Check sheet for the modelled part. Datum: model origin and axes. Units: mm. A direction names the side the tool comes from. Round coordinates to 2 decimals unless told otherwise and drop trailing zeros. Order: outer loops, then holes, each group sorted by start corner. A loop starts at its lowest first (then second) coordinate and runs counter-clockwise, first axis right, second up.
(1) Thickness scan on probe 1 along Y at (x, z) = (6.25, 8); probe 2 along Y at (x, z) = (-6.25, 5); probe 3 along X at (y, z) = (1, 5.75). Record the ranges inside material, lowest first.
(2) Mould release check, pull along Y, two halves, no side actions. Record for faces 1 (the cylindrical face through (11.25, -0.11, 8.73)), 2 (the cylindrical face through (-7.837, -1.217, 5.035)), 3 (the flat face through (3.8, 2.3, 7.5)): released by +Y, released by -Y, zero draft, split by the parting line, or undercut.
(3) Sectioned sample at D-D, the plane x = -1.5. Enter the section's corners in (y, z), and give its area (3 significant figures).
(4) Sectioned sample at C-C, the plane y = 3.75. Enter the section's corners in (x, z), and give its area (4 significant figures).
(5) Depth check by flat-ended pin: pin 1 (3.5 mm diameter, centred on x = 6.25, y = 0, fed in from -Z); pin 2 (1 mm diameter, centred on x = 8.5, y = -3.5, fed in from -Z); pin 3 (3 mm diameter, centred on y = 1.5, z = 1.5, fed in from -X); pin 4 (5 mm diameter, centred on x = 3.5, y = -1, fed in from -Z). Enter the tip coordinate at first touch or a pass-through.
(6) Sectioned sample at A-A, the plane y = 0. Enter the section's corners in (x, z), and give its area (3 significant figures).
(7) Sectioned sample at B-B, the plane z = 3.25. Enter the section's corners in (x, y), and give its area (3 significant figures).
(8) Tool access check on faces 4 (the flat face through (1.05, 0, 4)), 5 (the flat face through (-4, 0, 2.5)), 6 (the flat face through (-1.028, 0, 9)). Record the directions out of +Z, -Z, +X, -X, +Y, -Y that give a thin tool (end or side, any length) a straight path to the whole face; none if there is none.
```python
from build123d import *

# Parameters (mm, degrees)
EXTRUDE_1_DEPTH     = 10
SKETCH_3_W          = 5
SKETCH_3_H          = 2.5
CUT_EXTRUDE_2_DEPTH = 19.071040369
SKETCH_4_W          = 10.2
SKETCH_4_H          = 2.5
SKETCH_4_W_2        = 10.22157303
SKETCH_4_H_2        = 7.5
CUT_EXTRUDE_3_DEPTH = 19.071040369
EXTRUDE_START       = -1.5
SKETCH_2_R          = 2
EXTRUDE_2_DEPTH     = 3
SKETCH_2_3_R        = 3.1
SKETCH_2_3_R_2      = 2
CUT_EXTRUDE_4_DEPTH = 16.860721926


with BuildPart() as part:
    # Sketch 1 → Extrude 1 (new body)
    with BuildSketch(Plane.XY):
        with BuildLine():
            Line((-6.25, -5), (6.25, -5))
            ThreePointArc((6.25, -5), (11.25, 0), (6.25, 5))
            Line((6.25, 5), (-6.25, 5))
            ThreePointArc((-6.25, 5), (-11.25, 0), (-6.25, -5))
        make_face()
    extrude(amount=EXTRUDE_1_DEPTH)

    # Sketch 3 → Cut-Extrude 2 (cut, through all)
    with BuildSketch(Plane(origin=(0, 5, 0), x_dir=(1, 0, 0), z_dir=(0, 1, 0))):
        with Locations((8.75, -5)):
            Rectangle(SKETCH_3_W, SKETCH_3_H)
    extrude(amount=-CUT_EXTRUDE_2_DEPTH, mode=Mode.SUBTRACT)

    # Sketch 4 → Cut-Extrude 3 (cut, through all)
    with BuildSketch(Plane(origin=(0, 5, 0), x_dir=(1, 0, 0), z_dir=(0, 1, 0))):
        with Locations((-6.15, -1.25)):
            Rectangle(SKETCH_4_W, SKETCH_4_H)
        with Locations((-6.139213485, -8.75)):
            Rectangle(SKETCH_4_W_2, SKETCH_4_H)
        with Locations((6.15, -3.75)):
            Rectangle(SKETCH_4_W, SKETCH_4_H_2)
    extrude(amount=-CUT_EXTRUDE_3_DEPTH, mode=Mode.SUBTRACT)

    # Sketch 2 → Extrude 2 (add)
    with BuildSketch(Plane.XY.offset(10).offset(EXTRUDE_START)):
        with Locations((-6.25, 0)):
            Circle(SKETCH_2_R)
    extrude(amount=-EXTRUDE_2_DEPTH)

    # Sketch 2_3 → Cut-Extrude 4 (cut, through all)
    with BuildSketch(Plane.XY.offset(10)):
        with Locations((6.25, 0)):
            Circle(SKETCH_2_3_R)
        with Locations((-6.25, 0)):
            Circle(SKETCH_2_3_R_2)
    extrude(amount=-CUT_EXTRUDE_4_DEPTH, mode=Mode.SUBTRACT)


solid = part.part
```
Derived:
1. probe 1: y = -5 to -3.1, 3.1 to 5
1. probe 2: y = -5 to -2, 2 to 5
1. probe 3: x = -11.15 to -7.98, -4.52 to 1.05
2. face 1: split by the parting line
2. face 2: undercut
2. face 3: zero draft
3. outline: (-5, 2.5) - (5, 2.5) - (5, 7.5) - (-5, 7.5) - close
3. area: 50.0 mm2
4. outline: (-9.56, 2.5) - (-1.05, 2.5) - (-1.05, 0) - (1.05, 0) - (1.05, 7.5) - (9.56, 7.5) - (9.56, 10) - (-1.03, 10) - (-1.03, 7.5) - (-9.56, 7.5) - close
4. area: 84.75 mm2
5. pin 1: passes through
5. pin 2: stops at z = 7.5
5. pin 3: stops at x = -11.24
5. pin 4: stops at z = 0
6. outline: (-11.25, 2.5) - (-8.25, 2.5) - (-8.25, 7.5) - (-11.25, 7.5) - close; (-4.25, 2.5) - (-1.05, 2.5) - (-1.05, 0) - (1.05, 0) - (1.05, 7.5) - (3.15, 7.5) - (3.15, 10) - (-1.03, 10) - (-1.03, 7.5) - (-4.25, 7.5) - close; (9.35, 7.5) - (11.25, 7.5) - (11.25, 10) - (9.35, 10) - close
6. area: 61.9 mm2
7. outline: (-6.25, -5) - (1.05, -5) - (1.05, 5) - (-6.25, 5) arc R5 ccw to start; hole circle Ø4 at (-6.25, 0)
7. area: 99.7 mm2
8. face 4: -Z, +X, +Y, -Y
8. face 5: -Z, -X, +Y, -Y
8. face 6: +Z, -X, +Y, -Y
